Verification items for this drawing (mm, ordinates from the low corner). Round coordinates to 2 decimals unless told otherwise and drop trailing zeros. Loops run counter-clockwise (first coordinate to the right, second up) from the corner with the lowest first, then second, coordinate; pieces in that order, holes last. Notation, with made-up numbers: M 13,70.5 L 66,70.5 A31 ccw 66,109.5 Z; hole C 47.5,11 d8. An arc over 180 degrees is marked long. Answer in a Markdown table with one row per item. Add a question column.
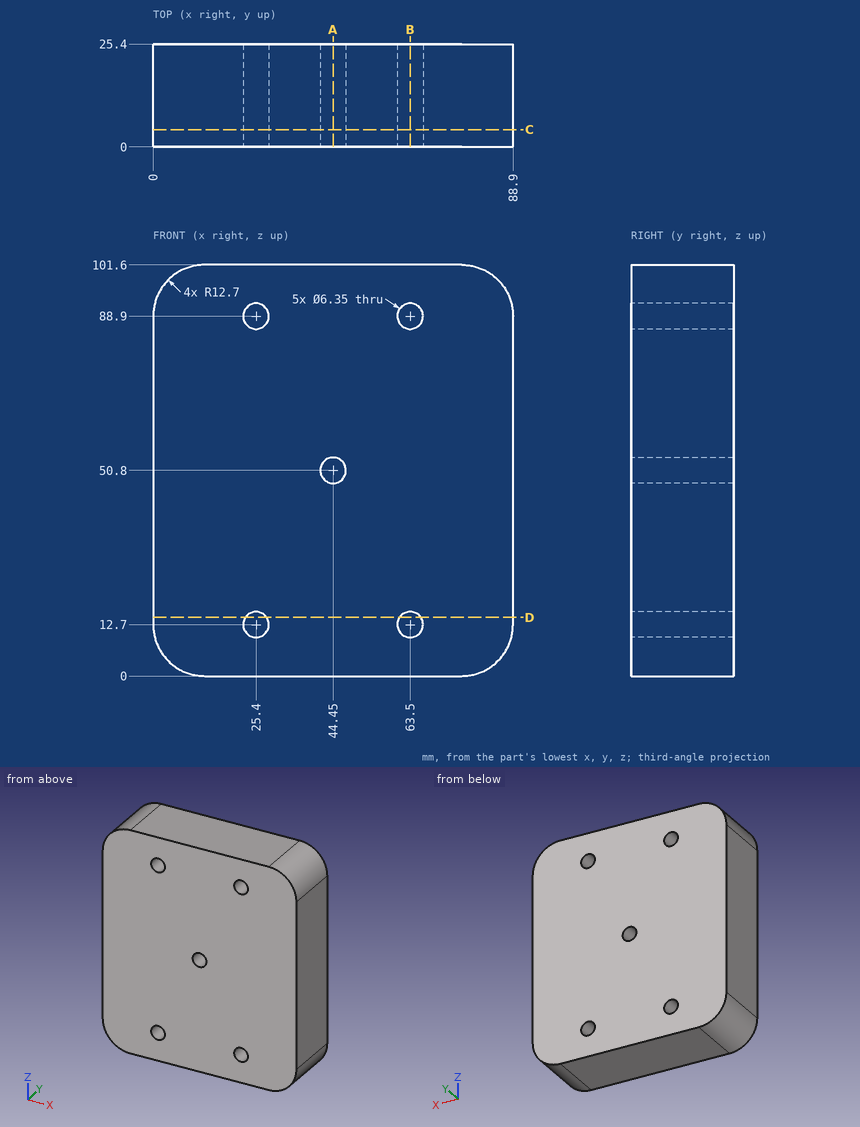
1) Cross-section at A-A, the plane x = 44.45. Record the boundary of the cut face in (y, z) (3 decimals).
2) Cross-section at B-B, the plane x = 63.5. Record the boundary of the cut face in (y, z) (3 decimals).
3) Cross-section at C-C, the plane y = 4.25. Record the boundary of the cut face in (x, z) (3 decimals).
4) Cross-section at D-D, the plane z = 14.5. Record the boundary of the cut face in (x, y).
5) Go/stop test with a flat-tipped pin: pin 1 (5 mm diameter, centred on x = 63.5, z = 12.7, fed in from +Y). Record where the tip stops, or that it passes through.
6) Thickness scan on L1, parallel to Z at x = 63.5, y = 5.5 (3 decimals); L2, parallel to X at y = 18, z = 12.7 (3 decimals); L3, parallel to X at y = 14.75, z = 88.5. Record the ranges inside material, lowest first. Write a range as [from, to].
Worked answers:
| question | item | result |
|---|---|---|
| 1 | outline | M 0,0 L 25.4,0 L 25.4,47.625 L 0,47.625 Z; M 0,53.975 L 25.4,53.975 L 25.4,101.6 L 0,101.6 Z |
| 2 | outline | M 0,0 L 25.4,0 L 25.4,9.525 L 0,9.525 Z; M 0,15.875 L 25.4,15.875 L 25.4,85.725 L 0,85.725 Z; M 0,92.075 L 25.4,92.075 L 25.4,101.6 L 0,101.6 Z |
| 3 | outline | M 0,12.7 A12.7 ccw 12.7,0 L 76.2,0 A12.7 ccw 88.9,12.7 L 88.9,88.9 A12.7 ccw 76.2,101.6 L 12.7,101.6 A12.7 ccw 0,88.9 Z; hole C 25.4,12.7 d6.35; hole C 25.4,88.9 d6.35; hole C 44.45,50.8 d6.35; hole C 63.5,12.7 d6.35; hole C 63.5,88.9 d6.35 |
| 4 | outline | M 0,0 L 22.78,0 L 22.78,25.4 L 0,25.4 Z; M 28.02,0 L 60.88,0 L 60.88,25.4 L 28.02,25.4 Z; M 66.12,0 L 88.9,0 L 88.9,25.4 L 66.12,25.4 Z |
| 5 | pin 1 | passes through |
| 6 | L1 | z = [0, 9.525], [15.875, 85.725], [92.075, 101.6] |
| 6 | L2 | x = [0, 22.225], [28.575, 60.325], [66.675, 88.9] |
| 6 | L3 | x = [0, 22.25], [28.55, 60.35], [66.65, 88.9] |
